from build123d import *

# Parameters (mm, degrees)
SKETCH1_R           = 50.8
BOSS_EXTRUDE1_DEPTH = 6.35
SKETCH4_R           = 50.8
SKETCH4_R_2         = 44.45
BOSS_EXTRUDE2_DEPTH = 19.05
SKETCH5_R           = 12.7
BOSS_EXTRUDE3_DEPTH = 19.05
CUT_EXTRUDE1_DEPTH  = 25.4


with BuildPart() as part:
    # Sketch1 → Boss-Extrude1 (new body)
    with BuildSketch(Plane(origin=(0, 0, 0), x_dir=(1, 0, 0), z_dir=(0, 1, 0))):
        with Locations(Location((0, 0, 0), (0, 0, 270))):
            Circle(SKETCH1_R)
    extrude(amount=BOSS_EXTRUDE1_DEPTH)

    # Sketch4 → Boss-Extrude2 (add)
    with BuildSketch(Plane(origin=(0, 6.35, 0), x_dir=(1, 0, 0), z_dir=(0, 1, 0))):
        with Locations(Location((0, 0, 0), (0, 0, 270))):
            Circle(SKETCH4_R)
        with Locations(Location((0, 0, 0), (0, 0, 90))):
            Circle(SKETCH4_R_2, mode=Mode.SUBTRACT)
    extrude(amount=BOSS_EXTRUDE2_DEPTH)

    # Sketch5 → Boss-Extrude3 (add)
    with BuildSketch(Plane(origin=(0, 6.35, 0), x_dir=(1, 0, 0), z_dir=(0, 1, 0))):
        with Locations(Location((0, 0, 0), (0, 0, 90))):
            Circle(SKETCH5_R)
    extrude(amount=BOSS_EXTRUDE3_DEPTH)

    # Sketch6 → Cut-Extrude1 (cut)
    with BuildSketch(Plane(origin=(0, 25.4, 0), x_dir=(1, 0, 0), z_dir=(0, 1, 0))):
        Polygon((-4.7625, -8.248891971), (4.7625, -8.248891971), (9.525, 0), (4.7625, 8.248891971), (-4.7625, 8.248891971), (-9.525, 0), align=None)
    extrude(amount=-CUT_EXTRUDE1_DEPTH, mode=Mode.SUBTRACT)


solid = part.part
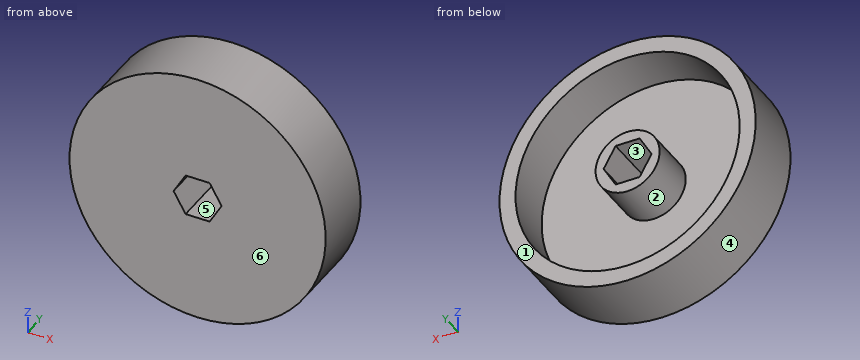
Read the model definition and answer for the solid it produces. Units are mm, in the model's axes. Face numbers are marked on the shaded views. A direction names the side the tool comes from. Coordinates: 2 decimals unless noted, no trailing zeros. Order: outer loops, then holes, each group sorted by start corner. A loop starts at its lowest first (then second) coordinate and runs counter-clockwise, first axis right, second up. Notation, with made-up numbers: (-6, 44.25) -> (37, 44.25) arc R30 ccw to (37, 81.25) -> close; hole circle Ø10 at (58, -11). An arc over 180 degrees is marked (long way). Answer as a JSON object with one key per item and string values.
1) The mould has two halves that part along X. Classify the marked faces 4, 5 and 6: released by +X, released by -X, zero draft, split by the parting line, or undercut.
Model answer:
{"face 4": "split by the parting line", "face 5": "undercut", "face 6": "zero draft"}
2) A tool of negligible diameter and unlimited length cuts with its end or side. For the marked faces 1, 2 and 3, from which of +Z, -Z, +X, -X, +Y, -Y can it reach the whole face along a straight path? Write none if from no direction.
Model answer:
{"face 1": "+Z, -Z, +X, -X, +Y", "face 2": "+Y", "face 3": "+Y, -Y"}
3) Each of these flat-tipped pins is pushed along its axis until it touches: pin 1 (3 mm diameter, centred on x = -9.5, y = 20.5, fed in from -Z); pin 2 (1.5 mm diameter, centred on y = 10, z = 28, fed in from -X); pin 3 (2 mm diameter, centred on x = 1.5, y = 17.5, fed in from -Z). Where does it stop, or does it pass through?
Model answer:
{"pin 1": "stops at z = -50.17", "pin 2": "stops at x = -42.87", "pin 3": "stops at z = -50.8"}
4) Consider line 1 along X through (y, z) = (13.75, 0) (3 decimals); line 2 along Z through (x, y) = (-4.5, 21.75); line 3 along Y through (x, z) = (25.5, -26). Determine where each line is inside the solid, lowest interval first. Write a range as from..to.
Model answer:
{"line 1": "x = -50.8..-44.45, -12.7..-9.525, 9.525..12.7, 44.45..50.8", "line 2": "z = -50.6..-44.22, -11.88..-8.25, 8.25..11.88, 44.22..50.6", "line 3": "y = 0..6.35"}
5) A cutting plane is placed at A-A, the plane y = 13. State how many separate pieces and enclosed holes the cut face has, plus the area to 3 significant figures.
Model answer:
{"separate pieces": "2", "enclosed holes": "2", "area": "2,170 mm²"}
6) A cutting plane is placed at C-C, the plane y = 2. Determine the outline of the cut face in (x, z) (1 decimal).
Model answer:
{"outline": "circle Ø101.6 at (0, 0); hole (-9.5, 0) -> (-4.8, -8.2) -> (4.8, -8.2) -> (9.5, 0) -> (4.8, 8.2) -> (-4.8, 8.2) -> close"}
7) A cutting plane is placed at B-B, the plane x = 0. Determine the outline of the cut face in (y, z), plus the area to 3 significant figures.
Model answer:
{"outline": "(0, -50.8) -> (25.4, -50.8) -> (25.4, -44.45) -> (6.35, -44.45) -> (6.35, -12.7) -> (25.4, -12.7) -> (25.4, -8.25) -> (0, -8.25) -> close; (0, 8.25) -> (25.4, 8.25) -> (25.4, 12.7) -> (6.35, 12.7) -> (6.35, 44.45) -> (25.4, 44.45) -> (25.4, 50.8) -> (0, 50.8) -> close", "area": "952 mm²"}
8) A cutting plane is placed at D-D, the plane z = -2. Determine the outline of the cut face in (x, y).
Model answer:
{"outline": "(-50.76, 0) -> (-8.37, 0) -> (-8.37, 25.4) -> (-12.54, 25.4) -> (-12.54, 6.35) -> (-44.4, 6.35) -> (-44.4, 25.4) -> (-50.76, 25.4) -> close; (8.37, 0) -> (50.76, 0) -> (50.76, 25.4) -> (44.4, 25.4) -> (44.4, 6.35) -> (12.54, 6.35) -> (12.54, 25.4) -> (8.37, 25.4) -> close"}
